Source: CAD feature listing. Evaluate the final solid. Frame: model axes, mm. Round coordinates to 2 decimals unless told otherwise and drop trailing zeros. Order: outer loops, then holes, each group sorted by start corner. A loop starts at its lowest first (then second) coordinate and runs counter-clockwise, first axis right, second up. Notation, with made-up numbers: (-11, 88) - (29, 88) arc R21 ccw to (29, 95) - close; hole circle Ø11 at (5.5, 50.25). An arc over 180 degrees is marked (long way). Put each result on its own line as item: value. Start each with the question number.
1) Contact query for a flat-ended pin moving along its axis: P1, Ø1, axis at y = -1, z = -83.5, coming from the -X side. Output: stop coordinate, or through.
2) Mould query, pull axis X, two halves, no side actions, for faces 1 (the face through (-31, -2.54, -41)), 2 (the face through (-16.89, -0.63, -23.43)), 3 (the face through (-16.998, -0.626, -84.572)). Classes: +X half, -X half, draft (parallel to the pull), parting line (faces both ways), or undercut.
3) Section C-C on y = -0.45. Output: boundary loops of the cut face in (x, z).
4) Line query: probe 1 along X at (y, z) = (-0.35, -10.5); probe 2 along X at (y, z) = (-2.1, 27). Output: solid intervals per line, ascending. Write a range as [from, to].
```python
from build123d import *

# Parameters (mm, degrees)
F1_DEPTH = 2.54
F2_SIZE  = 1.26999


# Not quite as in the source:
# - a fillet or chamfer is up to 0.001 mm smaller than in the source, because OpenCascade refuses the exact size


with BuildPart() as f1:
    # F0 (on Front) → F1 (new body)
    with BuildSketch(Plane.XZ):
        Polygon((20.5051476899, -109.5806663148), (-54.1552996701, 65.6793336852), (-54.1552996701, -61.3206663148), align=None)
    extrude(amount=F1_DEPTH)

    # F2 (size 1.27 in the source; OpenCascade refuses exactly that, so slightly less here)
    f2_edges = [f1.edges().sort_by_distance(p)[0] for p in [
        (-16.825076, -2.54, -85.450666),
        (-16.825076, -2.54, -21.950666),
        (-54.1553, -2.54, 2.179334),
        (-16.825076, 0, -85.450666),
        (-16.825076, 0, -21.950666),
        (-54.1553, 0, 2.179334),
    ]]
    chamfer(f2_edges, length=F2_SIZE)


solid = f1.part
```
Answer sheet:
1. P1: x = -20.49
2. face 1: draft
2. face 2: +X half
2. face 3: -X half
3. outline: (-53.34, -60.87) - (18.7, -107.44) - (-53.34, 61.66) - close
4. probe 1: [-53.24, -22.7]
4. probe 2: [-53.33, -38.58]
